from build123d import *

# Parameters (mm, degrees)
SKETCH1_R               = 3.5
BOSS_EXTRUDE1_DEPTH     = 1.5
BOSS_EXTRUDE2_DEPTH     = 3
SKETCH3_W               = 12
SKETCH3_H               = 12
SKETCH3_W_2             = 10
SKETCH3_H_2             = 10
BOSS_EXTRUDE3_DEPTH     = 0.7
SKETCH5_W               = 27.66
SKETCH5_H               = 27.66
CUT_EXTRUDE1_DEPTH      = 66.25114788
CUT_EXTRUDE2_DEPTH      = 66.25114788
CUT_EXTRUDE2_DEPTH_BACK = 1
SKETCH6_W               = 29.5
SKETCH6_H               = 31.81
CUT_EXTRUDE3_DEPTH      = 66.25114788
CUT_EXTRUDE3_DEPTH_BACK = 1
SKETCH4_W               = 14
SKETCH4_H               = 2.5
BOSS_EXTRUDE5_START     = -3
SKETCH8_W               = 1.5
SKETCH8_H               = 6
BOSS_EXTRUDE5_DEPTH     = 5


with BuildPart() as part:
    # Sketch1 → Boss-Extrude1 (new body)
    with BuildSketch(Plane(origin=(0, 0, 0), x_dir=(1, 0, 0), z_dir=(0, 1, 0))):
        with BuildLine():
            Line((0, -43.797867681), (0, -43))
            Line((0, -43), (0, -3))
            ThreePointArc((0, -3), (0.878679656, -0.878679656), (3, 0))
            Line((3, 0), (34, 0))
            ThreePointArc((34, 0), (36.121320344, -0.878679656), (37, -3))
            Line((37, -3), (37, -43))
            Line((37, -43), (37, -43.797867681))
            ThreePointArc((37, -43.797867681), (36.524802839, -45.925344888), (35.189536294, -47.648433643))
            ThreePointArc((35.189536294, -47.648433643), (18.5, -53.662950904), (1.810463706, -47.648433643))
            ThreePointArc((1.810463706, -47.648433643), (0.475197161, -45.925344888), (0, -43.797867681))
        make_face()
        with Locations(Location((27.28, -7.75, 0), (0, 0, 270))):
            Circle(SKETCH1_R, mode=Mode.SUBTRACT)
    extrude(amount=BOSS_EXTRUDE1_DEPTH)

    # Sketch2 → Boss-Extrude2 (add)
    with BuildSketch(Plane(origin=(0, 1.5, 0), x_dir=(1, 0, 0), z_dir=(0, 1, 0))):
        with BuildLine():
            Line((0, -43.797867681), (0, -43))
            Line((0, -43), (0, -3))
            ThreePointArc((0, -3), (0.878679656, -0.878679656), (3, 0))
            Line((3, 0), (34, 0))
            ThreePointArc((34, 0), (36.121320344, -0.878679656), (37, -3))
            Line((37, -3), (37, -43))
            Line((37, -43), (37, -43.797867681))
            ThreePointArc((37, -43.797867681), (36.524802839, -45.925344888), (35.189536294, -47.648433643))
            ThreePointArc((35.189536294, -47.648433643), (18.5, -53.662950904), (1.810463706, -47.648433643))
            ThreePointArc((1.810463706, -47.648433643), (0.475197161, -45.925344888), (0, -43.797867681))
        make_face()
        with BuildLine():
            Line((1.5, -43.797867681), (1.5, -43))
            Line((1.5, -43), (1.5, -4.5))
            ThreePointArc((1.5, -4.5), (2.378679656, -2.378679656), (4.5, -1.5))
            Line((4.5, -1.5), (32.5, -1.5))
            ThreePointArc((32.5, -1.5), (34.621320344, -2.378679656), (35.5, -4.5))
            Line((35.5, -4.5), (35.5, -43))
            Line((35.5, -43), (35.5, -43.797867681))
            ThreePointArc((35.5, -43.797867681), (35.167361988, -45.287101726), (34.232675406, -46.493263855))
            ThreePointArc((34.232675406, -46.493263855), (18.5, -52.162950904), (2.767324594, -46.493263855))
            ThreePointArc((2.767324594, -46.493263855), (1.832638012, -45.287101726), (1.5, -43.797867681))
        make_face(mode=Mode.SUBTRACT)
    extrude(amount=BOSS_EXTRUDE2_DEPTH)

    # Sketch3 → Boss-Extrude3 (add)
    with BuildSketch(Plane(origin=(0, 1.5, 0), x_dir=(1, 0, 0), z_dir=(0, 1, 0))):
        with Locations((27.28, -7.75)):
            Rectangle(SKETCH3_W, SKETCH3_H)
        with Locations((27.28, -7.75)):
            Rectangle(SKETCH3_W_2, SKETCH3_H_2, mode=Mode.SUBTRACT)
    extrude(amount=BOSS_EXTRUDE3_DEPTH)

    # Sketch5 → Cut-Extrude1 (cut, through all)
    with BuildSketch(Plane(origin=(0, 1.5, 0), x_dir=(1, 0, 0), z_dir=(0, 1, 0))):
        with Locations((18.48, -31.86)):
            Rectangle(SKETCH5_W, SKETCH5_H)
    extrude(amount=-CUT_EXTRUDE1_DEPTH, mode=Mode.SUBTRACT)

    # Sketch6 → Cut-Extrude2 (cut, two sides: drawn at the far end of the back side and taken through both)
    with BuildSketch(Plane(origin=(0, 1.5, 0), x_dir=(1, 0, 0), z_dir=(0, 1, 0)).offset(-CUT_EXTRUDE2_DEPTH_BACK)):
        with Locations((18.5, -30.885)):
            Rectangle(SKETCH6_W, SKETCH6_H)
    extrude(amount=CUT_EXTRUDE2_DEPTH + CUT_EXTRUDE2_DEPTH_BACK, mode=Mode.SUBTRACT)

    # Sketch4 → Cut-Extrude3 (cut, two sides: drawn at the far end of the back side and taken through both)
    with BuildSketch(Plane(origin=(0, 1.5, 0), x_dir=(1, 0, 0), z_dir=(0, 1, 0)).offset(-CUT_EXTRUDE3_DEPTH_BACK)):
        with Locations((18.48, -13.73)):
            Rectangle(SKETCH4_W, SKETCH4_H)
    extrude(amount=CUT_EXTRUDE3_DEPTH + CUT_EXTRUDE3_DEPTH_BACK, mode=Mode.SUBTRACT)

    # Sketch8 → Boss-Extrude5 (add)
    with BuildSketch(Plane(origin=(0, 4.5, 0), x_dir=(1, 0, 0), z_dir=(0, 1, 0)).offset(BOSS_EXTRUDE5_START)):
        with BuildLine():
            Line((1.5, -4.5), (1.5, -31.5))
            Line((1.5, -31.5), (3, -31.5))
            Line((3, -31.5), (3, -4.5))
            ThreePointArc((3, -4.5), (3.439339828, -3.439339828), (4.5, -3))
            Line((4.5, -3), (18.5, -3))
            Line((18.5, -3), (18.5, -1.5))
            Line((18.5, -1.5), (4.5, -1.5))
            ThreePointArc((4.5, -1.5), (2.378679656, -2.378679656), (1.5, -4.5))
        make_face()
        with Locations((34.75, -28.5)):
            Rectangle(SKETCH8_W, SKETCH8_H)
        with BuildLine():
            Line((35.5, -43), (35.5, -43.797867681))
            ThreePointArc((35.5, -43.797867681), (35.167361988, -45.287101726), (34.232675406, -46.493263855))
            ThreePointArc((34.232675406, -46.493263855), (18.5, -52.162950904), (2.767324594, -46.493263855))
            ThreePointArc((2.767324594, -46.493263855), (1.832638012, -45.287101726), (1.5, -43.797867681))
            Line((1.5, -43.797867681), (1.5, -43))
            Line((1.5, -43), (1.5, -39.5))
            Line((1.5, -39.5), (3, -39.5))
            Line((3, -39.5), (3, -43))
            Line((3, -43), (3, -43.797867681))
            ThreePointArc((3, -43.797867681), (3.190078864, -44.648858564), (3.724185482, -45.338094066))
            ThreePointArc((3.724185482, -45.338094066), (18.5, -50.662950904), (33.275814518, -45.338094066))
            ThreePointArc((33.275814518, -45.338094066), (33.809921136, -44.648858564), (34, -43.797867681))
            Line((34, -43.797867681), (34, -43))
            Line((34, -43), (34, -39.5))
            Line((34, -39.5), (35.5, -39.5))
            Line((35.5, -39.5), (35.5, -43))
        make_face()
    extrude(amount=BOSS_EXTRUDE5_DEPTH)


solid = part.part
Work out the finished part from the listing and answer in its coordinate system (mm). A direction names the side the tool comes from. Give positions to 0.01 mm unless a question says otherwise; leave off trailing zeros. Loops run counter-clockwise (first coordinate to the right, second up) from the corner with the lowest first, then second, coordinate; pieces in that order, holes last. Notation, with made-up numbers: (15, -29) -> (68, -29) arc R31 cw to (68, 8) -> close; hole circle Ø11 at (85, 3). An arc over 180 degrees is marked (long way). Use a Markdown table: item, result. Add a question column.
1) Each of these flat-tipped pins is pushed along its axis until it touches: P1, Ø11, axis at x = 28.5, z = 6.5, coming from the +Y side; P2, Ø2.5, axis at x = 26, y = 3, coming from the +Z side; P3, Ø1.9, axis at x = 23.5, z = 48, coming from the +Y side. Where does it stop, or does it pass through?
2) Consider line 1 along X through (y, z) = (0.4, 7.75); line 2 along X through (y, z) = (2.5, 29); line 3 along Z through (x, y) = (24.5, 1.25). Determine where each line is inside the solid, lowest interval first.
3) Which of the six approach directions +Z, -Z, +X, -X, +Y, -Y give full straight-line access (tool end or side, diameter ignored) to faces 1 (the flat face through (35.5, 5, 29)), 2 (the flat face through (34, 4, 42)), 3 (the flat face through (19, 0, 15))?
4) The part is cut by section D-D, the plane z = 38.5. Determine the outline of the cut face in (x, y), plus the area to 3 significant figures.
5) For a pull along Z with two mould halves and no side action, classify faces 4 (the cylindrical face through (1.842, 5.486, 45.307)), 5 (the cylindrical face through (36.1, 2.22, 0.86)), 6 (the flat face through (36, 4.5, 23)), 7 (the flat face through (11, 4, 3)) as +Z half, -Z half, draft (parallel to the pull), parting line (faces both ways), or undercut.
6) The part is cut by section A-A, the plane z = 7.75. Determine the outline of the cut face in (x, y), plus the area to 3 significant figures.
7) The part is cut by section B-B, the plane x = 27.28. Count the separate pieces of the cut face and the enclosed holes in it, plus the area to 3 significant figures.
8) The part is cut by section C-C, the plane x = 10.5. Determine the outline of the cut face in (y, z), plus the area to 3 significant figures.
Reported:
| question | item | result |
|---|---|---|
| 1 | P1 | stops at y = 4.5 |
| 1 | P2 | stops at z = 52.91 |
| 1 | P3 | stops at y = 1.5 |
| 2 | line 1 | x = 0 to 23.78, 30.78 to 37 |
| 2 | line 2 | x = 0 to 3, 34 to 37 |
| 2 | line 3 | z = 0 to 5.62, 9.88 to 12.48, 46.79 to 52.97 |
| 3 | face 1 | +Z, -Z, +X, +Y |
| 3 | face 2 | +Y |
| 3 | face 3 | +Z, -Z, +X, -X, -Y |
| 4 | outline | (0, 0) -> (4.65, 0) -> (4.65, 0.5) -> (3.75, 0.5) -> (3.75, 1.5) -> (1.5, 1.5) -> (1.5, 4.5) -> (0, 4.5) -> close; (32.31, 0) -> (37, 0) -> (37, 4.5) -> (35.5, 4.5) -> (35.5, 1.5) -> (33.25, 1.5) -> (33.25, 0.5) -> (32.31, 0.5) -> close |
| 4 | area | 21.2 mm^2 |
| 5 | face 4 | +Z half |
| 5 | face 5 | -Z half |
| 5 | face 6 | draft |
| 5 | face 7 | undercut |
| 6 | outline | (0, 0) -> (23.78, 0) -> (23.78, 1.5) -> (22.28, 1.5) -> (22.28, 2.2) -> (21.28, 2.2) -> (21.28, 1.5) -> (3, 1.5) -> (3, 6.5) -> (1.5, 6.5) -> (1.5, 4.5) -> (0, 4.5) -> close; (30.78, 0) -> (37, 0) -> (37, 4.5) -> (35.5, 4.5) -> (35.5, 1.5) -> (33.28, 1.5) -> (33.28, 2.2) -> (32.28, 2.2) -> (32.28, 1.5) -> (30.78, 1.5) -> close |
| 6 | area | 62.9 mm^2 |
| 7 | separate pieces | 3 |
| 7 | enclosed holes | 0 |
| 7 | area | 40.8 mm^2 |
| 8 | outline | (0, 0) -> (4.5, 0) -> (4.5, 1.5) -> (6.5, 1.5) -> (6.5, 3) -> (1.5, 3) -> (1.5, 14.98) -> (0.5, 14.98) -> (0.5, 18.03) -> (0, 18.03) -> close; (0, 45.69) -> (0.5, 45.69) -> (0.5, 46.79) -> (1.5, 46.79) -> (1.5, 49.24) -> (6.5, 49.24) -> (6.5, 50.83) -> (4.5, 50.83) -> (4.5, 52.41) -> (0, 52.41) -> close |
| 8 | area | 57.7 mm^2 |
